For this review, take the finished solid that the model builds, in its own axes (mm). A direction names the side the tool comes from. Give positions to 0.01 mm unless a question says otherwise; leave off trailing zeros. Loops run counter-clockwise (first coordinate to the right, second up) from the corner with the lowest first, then second, coordinate; pieces in that order, holes last. Notation, with made-up numbers: (-12.75, 12) - (31.25, 12) arc R16 cw to (31.25, 30) - close; hole circle Ø6 at (-34.5, -7.5). An arc over 180 degrees is marked (long way). Answer in a Markdown table with one row per item.
```python
from build123d import *

# Parameters (mm, degrees)
CROQUIS3_R              = 12.5
CROQUIS3_R_2            = 6
CROQUIS3_R_3            = 5
SALIENTE_EXTRUIR1_DEPTH = 15
SALIENTE_EXTRUIR2_START = 15
CROQUIS4_R              = 7.5
SALIENTE_EXTRUIR2_DEPTH = 2
SALIENTE_EXTRUIR3_DEPTH = 40
CROQUIS6_R              = 22.5
CROQUIS6_R_2            = 6
SALIENTE_EXTRUIR4_DEPTH = 25


with BuildPart() as part:
    # Croquis3 → Saliente-Extruir1 (new body)
    with BuildSketch(Plane(origin=(0, 0, 0), x_dir=(1, 0, 0), z_dir=(0, 1, 0))):
        with BuildLine():
            Line((60, 50), (-60, 50))
            ThreePointArc((-60, 50), (-70.606601718, 45.606601718), (-75, 35))
            Line((-75, 35), (-75, -35))
            ThreePointArc((-75, -35), (-70.606601718, -45.606601718), (-60, -50))
            Line((-60, -50), (60, -50))
            ThreePointArc((60, -50), (70.606601718, -45.606601718), (75, -35))
            Line((75, -35), (75, 35))
            ThreePointArc((75, 35), (70.606601718, 45.606601718), (60, 50))
        make_face()
        with Locations(Location((0, 0, 0), (0, 0, 270))):
            Circle(CROQUIS3_R, mode=Mode.SUBTRACT)
        with Locations(Location((-28, -28, 0), (0, 0, 270))):
            Circle(CROQUIS3_R_2, mode=Mode.SUBTRACT)
        with Locations(Location((-28, 28, 0), (0, 0, 270))):
            Circle(CROQUIS3_R_2, mode=Mode.SUBTRACT)
        with Locations(Location((28, 28, 0), (0, 0, 270))):
            Circle(CROQUIS3_R_2, mode=Mode.SUBTRACT)
        with Locations(Location((60, 35, 0), (0, 0, 270))):
            Circle(CROQUIS3_R_3, mode=Mode.SUBTRACT)
        with Locations(Location((60, -35, 0), (0, 0, 270))):
            Circle(CROQUIS3_R_3, mode=Mode.SUBTRACT)
        with Locations(Location((-60, -35, 0), (0, 0, 270))):
            Circle(CROQUIS3_R_3, mode=Mode.SUBTRACT)
        with Locations(Location((-60, 35, 0), (0, 0, 270))):
            Circle(CROQUIS3_R_3, mode=Mode.SUBTRACT)
    extrude(amount=SALIENTE_EXTRUIR1_DEPTH)

    # Croquis4 → Saliente-Extruir2 (add)
    with BuildSketch(Plane(origin=(0, 0, 0), x_dir=(1, 0, 0), z_dir=(0, 1, 0)).offset(SALIENTE_EXTRUIR2_START)):
        with Locations((60, -35)):
            Circle(CROQUIS4_R)
        with Locations((60, 35)):
            Circle(CROQUIS4_R)
        with Locations((-60, 35)):
            Circle(CROQUIS4_R)
        with Locations((-60, -35)):
            Circle(CROQUIS4_R)
    extrude(amount=-SALIENTE_EXTRUIR2_DEPTH)

    # Croquis5 → Saliente-Extruir3 (add)
    with BuildSketch(Plane(origin=(0, 0, 0), x_dir=(1, 0, 0), z_dir=(0, 1, 0))):
        with BuildLine():
            Line((50, -35), (50, 35))
            ThreePointArc((50, 35), (45.606601718, 45.606601718), (35, 50))
            Line((35, 50), (-35, 50))
            ThreePointArc((-35, 50), (-45.606601718, 45.606601718), (-50, 35))
            Line((-50, 35), (-50, -35))
            ThreePointArc((-50, -35), (-45.606601718, -45.606601718), (-35, -50))
            Line((-35, -50), (35, -50))
            ThreePointArc((35, -50), (45.606601718, -45.606601718), (50, -35))
        make_face()
        with BuildLine():
            Line((35, 40), (-35, 40))
            ThreePointArc((-35, 40), (-38.535533906, 38.535533906), (-40, 35))
            Line((-40, 35), (-40, -35))
            ThreePointArc((-40, -35), (-38.535533906, -38.535533906), (-35, -40))
            Line((-35, -40), (35, -40))
            ThreePointArc((35, -40), (38.535533906, -38.535533906), (40, -35))
            Line((40, -35), (40, 35))
            ThreePointArc((40, 35), (38.535533906, 38.535533906), (35, 40))
        make_face(mode=Mode.SUBTRACT)
    extrude(amount=SALIENTE_EXTRUIR3_DEPTH)

    # Croquis6 → Saliente-Extruir4 (add)
    with BuildSketch(Plane(origin=(0, 0, 0), x_dir=(1, 0, 0), z_dir=(0, 1, 0))):
        with BuildLine():
            Line((-35, -40), (35, -40))
            ThreePointArc((35, -40), (38.535533906, -38.535533906), (40, -35))
            Line((40, -35), (40, 35))
            ThreePointArc((40, 35), (38.535533906, 38.535533906), (35, 40))
            Line((35, 40), (-35, 40))
            ThreePointArc((-35, 40), (-38.535533906, 38.535533906), (-40, 35))
            Line((-40, 35), (-40, -35))
            ThreePointArc((-40, -35), (-38.535533906, -38.535533906), (-35, -40))
        make_face()
        with Locations(Location((0, 0, 0), (0, 0, 270))):
            Circle(CROQUIS6_R, mode=Mode.SUBTRACT)
        with Locations(Location((28, 28, 0), (0, 0, 270))):
            Circle(CROQUIS6_R_2, mode=Mode.SUBTRACT)
        with Locations(Location((28, -28, 0), (0, 0, 270))):
            Circle(CROQUIS6_R_2, mode=Mode.SUBTRACT)
        with Locations(Location((-28, -28, 0), (0, 0, 270))):
            Circle(CROQUIS6_R_2, mode=Mode.SUBTRACT)
        with Locations(Location((-28, 28, 0), (0, 0, 270))):
            Circle(CROQUIS6_R_2, mode=Mode.SUBTRACT)
    extrude(amount=SALIENTE_EXTRUIR4_DEPTH)


solid = part.part
```
1. For faces 1 (the face through (50, 27, 0)), 2 (the face through (39, 32, -38)), 3 (the face through (63, 6, 31)), list the 3-axis set-ups (+Z, -Z, +X, -X, +Y, -Y) from which the entire face can be reached by the end or side of a thin tool; tool diameter is ignored.
Values:
| item | result |
|---|---|
| face 1 | +Z, -Z, +X, +Y |
| face 2 | +Y |
| face 3 | -Y |
2. Mouldability with a two-part tool opening along Z and no side actions: class faces 4 (the face through (-40, 32, 0)), 5 (the face through (16, 0, -1)), 6 (the face through (45.49, 27.32, 45.72)), 7 (the face through (17, 25, -18)) as released by +Z, released by -Z, zero draft, split by the parting line, or undercut.
Values:
| item | result |
|---|---|
| face 4 | undercut |
| face 5 | zero draft |
| face 6 | released by +Z |
| face 7 | undercut |
3. Wall thickness on line 1 (X direction, y = 7, z = 35); line 2 (X direction, y = 7, z = 0); line 3 (Z direction, x = 28, y = 37.5): over which ranges is each line inside the solid? List them lowest first. Write a range as [from, to].
Values:
| item | result |
|---|---|
| line 1 | x = [-75, -65], [-55, 55], [65, 75] |
| line 2 | x = [-75, -12.5], [12.5, 75] |
| line 3 | z = [-50, -40], [40, 50] |
4. We need section C-C, the plane y = 17. Give the boundary of the cut face in (x, z), and give its area (3 significant figures).
Values:
| item | result |
|---|---|
| outline | (-50, -35) arc R15 ccw to (-35, -50) - (35, -50) arc R15 ccw to (50, -35) - (50, 35) arc R15 ccw to (35, 50) - (-35, 50) arc R15 ccw to (-50, 35) - close; hole circle Ø12 at (-28, -28); hole circle Ø12 at (-28, 28); hole circle Ø45 at (0, 0); hole circle Ø12 at (28, -28); hole circle Ø12 at (28, 28) |
| area | 7,760 mm^2 |
5. Clearance check with flat-ended pins moving along their axes: pin 1 (5 mm diameter, centred on x = 59.5, z = 33, fed in from -Y); pin 2 (1.5 mm diameter, centred on x = -40.5, y = 31, fed in from -Z); pin 3 (7.5 mm diameter, centred on y = 34.5, z = -3, fed in from -X). State where each tip first meets the part, or that it passes through.
Values:
| item | result |
|---|---|
| pin 1 | stops at y = 13 |
| pin 2 | stops at z = -49.23 |
| pin 3 | stops at x = -50 |
6. We need section D-D, the plane z = -28. Give the boundary of the cut face in (x, y).
Values:
| item | result |
|---|---|
| outline | (-75, 0) - (-34, 0) - (-34, 25) - (-40, 25) - (-40, 40) - (-50, 40) - (-50, 15) - (-75, 15) - close; (-22, 0) - (22, 0) - (22, 25) - (-22, 25) - close; (34, 0) - (75, 0) - (75, 15) - (50, 15) - (50, 40) - (40, 40) - (40, 25) - (34, 25) - close |
7. We need section B-B, the plane x = 28. Give the boundary of the cut face in (y, z), and give its area (3 significant figures).
Values:
| item | result |
|---|---|
| outline | (0, -50) - (40, -50) - (40, -40) - (25, -40) - (25, -34) - (0, -34) - close; (0, -22) - (25, -22) - (25, 22) - (15, 22) - (15, 34) - (25, 34) - (25, 40) - (40, 40) - (40, 50) - (0, 50) - close |
| area | 2,380 mm^2 |
8. We need section A-A, the plane z = 0. Give the boundary of the cut face in (x, y).
Values:
| item | result |
|---|---|
| outline | (-75, 0) - (-12.5, 0) - (-12.5, 15) - (-22.5, 15) - (-22.5, 25) - (-40, 25) - (-40, 40) - (-50, 40) - (-50, 15) - (-75, 15) - close; (12.5, 0) - (75, 0) - (75, 15) - (50, 15) - (50, 40) - (40, 40) - (40, 25) - (22.5, 25) - (22.5, 15) - (12.5, 15) - close |
